```python
from build123d import *

# Parameters (mm, degrees)
F1_DEPTH      = 19.05
F1_DEPTH_BACK = 19.05
F2_R          = 8.7708682623
F4_DEPTH      = 3.81
F5_SIZE       = 0.254
F6_R          = 8.5644348715
F7_DEPTH      = 131.826
F8_R          = 7.62


with BuildPart() as f1:
    # F0 (on Right) → F1 (new body, two sides)
    with BuildSketch(Plane.YZ) as f1_sk:
        with BuildLine():
            ThreePointArc((-69.297126121, 10.6023983714), (-90.5654400371, -9.9203811878), (-117.0916636607, -22.9543797277))
            Line((-117.0916636607, -22.9543797277), (86.1083363393, -19.6213065932))
            Line((86.1083363393, -19.6213065932), (43.3460188102, 0))
            Line((43.3460188102, 0), (-69.297126121, 10.6023983714))
        make_face()
    extrude(amount=F1_DEPTH)
    extrude(f1_sk.sketch, amount=-F1_DEPTH_BACK)

    # F2
    f2_edges = [f1.edges().sort_by_distance(p)[0] for p in [
        (0, -69.297126, 10.602398),
    ]]
    fillet(f2_edges, radius=F2_R)

    # F3 (on face) → F4 (join)
    with BuildSketch(Plane(origin=(0, 0.380642539, 4.0440635396), x_dir=(1, 0, 0), z_dir=(0, 0.0937095933, 0.9955995742))):
        Polygon((-76.7426812672, 17.75527787), (0, -60.1567947547), (0, 17.75527787), align=None)
        Polygon((0, 17.75527787), (0, -60.1567947547), (76.2, 17.75527787), align=None)
    extrude(amount=-F4_DEPTH)

    # F5
    f5_edges = [f1.edges().sort_by_distance(p)[0] for p in [
        (47.625, -11.387704, 1.324905),
        (47.625, -11.03067, 5.118139),
        (-47.896341, -11.099236, 5.124593),
        (-47.896341, -11.45627, 1.331359),
    ]]
    chamfer(f5_edges, length=F5_SIZE)

    # F6 (on Front) → F7 (cut)
    with BuildSketch(Plane.XZ):
        with Locations((0, -8.5168717217)):
            Circle(F6_R)
    extrude(amount=-F7_DEPTH, mode=Mode.SUBTRACT)

    # F8
    f8_edges = [f1.edges().sort_by_distance(p)[0] for p in [
        (-8.564435, 0, -8.516872),
    ]]
    fillet(f8_edges, radius=F8_R)


solid = f1.part
```
Design review of the part built by this model. Coordinates are the model's own, in mm. A direction names the side the tool comes from. Coordinates: 2 decimals unless noted, no trailing zeros. Order: outer loops, then holes, each group sorted by start corner. A loop starts at its lowest first (then second) coordinate and runs counter-clockwise, first axis right, second up.
1) Clearance check with flat-ended pins moving along their axes: pin 1 (10 mm diameter, centred on y = -40.5, z = -7.5, fed in from -X); pin 2 (12 mm diameter, centred on x = 25.5, z = -15, fed in from +Y); pin 3 (0.6 mm diameter, centred on x = -0.5, z = -8.5, fed in from +Y); pin 4 (6 mm diameter, centred on x = 18, z = -11.5, fed in from +Y). State where each tip first meets the part, or that it passes through.
2) Mouldability with a two-part tool opening along X and no side actions: class faces 4 (the cylindrical face through (0.27, -92.12, -10.99)), 5 (the flat face through (47.23, -11.27, 5.01)), 6 (the flat face through (-48.3, -10.87, 3.21)), 7 (the cylindrical face through (-1.857, 35.48, -16.878)) as +X half, -X half, draft (parallel to the pull), parting line (faces both ways), or undercut.
3) Take a section at A-A, the plane x = -14. Give the boundary of the cut face in (y, z).
4) Take a section at B-B, the plane y = -46.5. Give the boundary of the cut face in (x, z).
5) Wall thickness on line 1 along X through (y, z) = (44, -8.5); line 2 along X through (y, z) = (36, -8); line 3 along X through (y, z) = (-24.5, -18): over which ranges is each line inside the solid? List them lowest first.
6) For faces 1 (the flat face through (-35.378, 2.008, 0.064)), 2 (the flat face through (47.225, -11.614, 3.283)), 3 (the flat face through (40.739, -4.378, 0.665)), list the 3-axis set-ups (+Z, -Z, +X, -X, +Y, -Y) from which the entire face can be reached by the end or side of a thin tool; tool diameter is ignored.
Returned:
1. pin 1: stops at x = -19.05
1. pin 2: passes through
1. pin 3: stops at y = 0
1. pin 4: stops at y = 74.95
2. face 4: draft
2. face 5: +X half
2. face 6: -X half
2. face 7: undercut
3. outline: (-117.09, -22.95) - (86.11, -19.62) - (43.35, 0) - (-64.57, 10.16) arc R8.77 ccw to (-72.13, 7.04) arc R95.46 cw to start
4. outline: (-19.05, -21.8) - (19.05, -21.8) - (19.05, 8.46) - (-19.05, 8.46) - close
5. line 1: x = -19.05 to -8.56, 8.56 to 19.05
5. line 2: x = -19.05 to -8.55, 8.55 to 19.05
5. line 3: x = -19.05 to 19.05
6. face 1: -Z, -X, -Y
6. face 2: +Z, +X, -Y
6. face 3: -Z, +X, -Y
